Part model, mm, in its own coordinate system. A direction names the side the tool comes from. Round coordinates to 2 decimals unless told otherwise and drop trailing zeros. Write each loop counter-clockwise with the first axis right and the second up, starting at its lowest first coordinate (ties: lowest second). Pieces come first, ordered by that corner, then holes. Notation, with made-up numbers: M 6.25,-16.75 L 21.25,-16.75 A9 cw 21.25,-10.75 Z; hole C -10,63.5 d5. An arc over 180 degrees is marked long. Use a Markdown table: item, result. Add a question column.
1) Slice it at A-A on y = -4.25. Write the cut outline in (x, z).
2) Two-plate mould, pull along Z, no slides. Class faces 1 (the face through (-2.278, 1.597, -1.746)), 2 (the face through (0.111, 1.219, -0.213)), 3 (the face through (0, 3.505, -2)): released by +Z, released by -Z, zero draft, split by the parting line, or undercut.
3) Drop flat-ended pins along their axis: P1, Ø1, axis at y = 2, z = 1, coming from the -X side; P2, Ø1, axis at y = -5, z = -1.5, coming from the +X side; P3, Ø2, axis at y = -3, z = 0, coming from the +X side. Give the stop position or say it passes through.
4) Which spindle directions (+Z, -Z, +X, -X, +Y, -Y) get a long thin tool onto all of the face, cutting with end or side? Do faces 4 (the face through (1.204, 2.704, -0.682)), 5 (the face through (1.67, -3.03, 0.53)), 6 (the face through (0, -6.35, 0)). Say none if no direction does.
5) Wall check: probe 1 along Z at (x, y) = (0, 2.5); probe 2 along Z at (x, y) = (0.05, -2.25); probe 3 along Y at (x, z) = (1.3, 1.75). Give the ranges that are in metal, low to high.
```python
from build123d import *

# Parameters (mm, degrees)
SKETCH1_W           = 2.8702
SKETCH1_H           = 3.5052
SKETCH2_R           = 1.7526
BOSS_EXTRUDE1_DEPTH = 6.35
CUT_EXTRUDE1_DEPTH  = 1.6256
CHAMFER1_SIZE       = 0.47244
CHAMFER2_SIZE       = 0.3556
FILLET1_R           = 0.254


with BuildPart() as part:
    # Sketch1 → Revolve1 (revolve)
    with BuildSketch(Plane.XY):
        with Locations((1.4351, 1.7526)):
            Rectangle(SKETCH1_W, SKETCH1_H)
    revolve(axis=Axis((0, 3.5052, 0), (0, -1, 0)))

    # Sketch2 → Boss-Extrude1 (add)
    with BuildSketch(Plane.XZ):
        Circle(SKETCH2_R)
    extrude(amount=BOSS_EXTRUDE1_DEPTH)

    # Sketch3 → Cut-Extrude1 (cut)
    with BuildSketch(Plane(origin=(0, 3.5052, 0), x_dir=(-1, 0, 0), z_dir=(0, 1, 0))):
        Polygon((-1.598451955, 0), (-0.799225978, -1.3843), (0.799225978, -1.3843), (1.598451955, 0), (0.799225978, 1.3843), (-0.799225978, 1.3843), align=None)
    extrude(amount=-CUT_EXTRUDE1_DEPTH, mode=Mode.SUBTRACT)

    # Sketch4 → Cut-Revolve1 (revolve, cut)
    with BuildSketch(Plane.XY):
        Polygon((1.3843, 1.8796), (0, 1.8796), (0, 1.080374022), align=None)
    revolve(axis=Axis((0, 1.8796, 0), (0, -1, 0)), mode=Mode.SUBTRACT)

    # Chamfer1
    chamfer1_edges = [part.edges().sort_by_distance(p)[0] for p in [
        (-1.7526, -6.35, 0),
    ]]
    chamfer(chamfer1_edges, length=CHAMFER1_SIZE)

    # Chamfer2
    chamfer2_edges = [part.edges().sort_by_distance(p)[0] for p in [
        (-2.8702, 3.5052, 0),
    ]]
    chamfer(chamfer2_edges, length=CHAMFER2_SIZE)

    # Fillet1
    fillet1_edges = [part.edges().sort_by_distance(p)[0] for p in [
        (-1.7526, 0, 0),
    ]]
    fillet(fillet1_edges, radius=FILLET1_R)


solid = part.part
```
Entries:
| question | item | result |
|---|---|---|
| 1 | outline | C 0,0 d3.51 |
| 2 | face 1 | split by the parting line |
| 2 | face 2 | undercut |
| 2 | face 3 | zero draft |
| 3 | P1 | stops at x = -2.83 |
| 3 | P2 | stops at x = 1.44 |
| 3 | P3 | stops at x = 1.75 |
| 4 | face 4 | +Y |
| 4 | face 5 | -Y |
| 4 | face 6 | +Z, -Z, +X, -X, -Y |
| 5 | probe 1 | z = -2.87 to -1.38, 1.38 to 2.87 |
| 5 | probe 2 | z = -1.75 to 1.75 |
| 5 | probe 3 | y = 0 to 3.51 |
